Source: CAD feature listing. Evaluate the final solid. Frame: model axes, mm. A direction names the side the tool comes from. Give positions to 0.01 mm unless a question says otherwise; leave off trailing zeros. Write each loop counter-clockwise with the first axis right and the second up, starting at its lowest first coordinate (ties: lowest second). Pieces come first, ordered by that corner, then holes. Notation, with made-up numbers: (9, 66.25) -> (62, 66.25) arc R20 ccw to (62, 98.25) -> close; hole circle Ø9 at (-35.75, 40.25). An arc over 180 degrees is marked (long way). Answer as a JSON object with one key per item and string values. Group by question number.
Item 1: Pull-direction query (X, two-part tool) for faces 4 (the face through (-1.42, -3.92, 0)), 5 (the face through (-0.867, -3.905, 6.902)), 6 (the face through (1, -1, 7)); classes: pulls with the +X half, pulls with the -X half, needs draft (parallel to the pull), parting line crosses it, or undercut.
Item 2: Section query B-B on y = 0. Return the cut outline in (x, z).
Item 3: First-contact query: pin 1 Ø3 at (x, z) = (0, 7.5) entering from -Y; pin 2 Ø6 at (x, z) = (2.5, 7) entering from +Y; pin 3 Ø2 at (x, z) = (-4.5, 11.5) entering from -Y. Flat tips, straight axial feed; report the tip coordinate or a pass-through.
Item 4: Section query A-A on x = 0. Return the cut outline in (y, z).
Item 5: Section query C-C on z = 13.25. Return the cut outline in (x, y).
Item 6: Ray query, probe 1 along Y at (x, z) = (0, 12.5); probe 2 along Y at (x, z) = (-0.5, 10); probe 3 along Z at (x, y) = (3.5, -4). Return the intervals inside material, ascending. Write a range as from..to.
Item 7: Section query D-D on z = 3.5. Return the cut outline in (x, y), plus the area to 3 significant figures.
Item 8: Access query for faces 1 (the face through (4.197, 1.322, 14.394)), 2 (the face through (-0.06, -1.7, 2.94)), 3 (the face through (-0.1, 1.4, -1)). Directions: +Z, -Z, +X, -X, +Y, -Y. A direction counts if a zero-diameter tool reaches every point of the face in a straight line with its end or side. Return the directions, or none.
from build123d import *

# Parameters (mm, degrees)
SKETCH_R             = 4
PAD_DEPTH            = 14
SKETCH001_R          = 4.4
PAD001_DEPTH         = 1.5
CHAMFER_SIZE         = 0.7
SKETCH002_R          = 6
PAD002_DEPTH         = 1
POCKET_DEPTH         = 8
SKETCH004_R          = 1
POCKET001_DEPTH      = 1.001
POCKET001_DEPTH_BACK = -15.501


with BuildPart() as part:
    # Sketch → Pad (new body)
    with BuildSketch(Plane.XY):
        Circle(SKETCH_R)
    extrude(amount=PAD_DEPTH)

    # Sketch001 (on Face3 of Pad) → Pad001 (join)
    with BuildSketch(Plane.XY.offset(14)):
        Circle(SKETCH001_R)
    extrude(amount=PAD001_DEPTH)

    # Chamfer
    chamfer_edges = [part.edges().sort_by_distance(p)[0] for p in [
        (-4.4, 0, 15.5),
    ]]
    chamfer(chamfer_edges, length=CHAMFER_SIZE)

    # Sketch002 → Pad002 (join)
    with BuildSketch(Plane.XY):
        Circle(SKETCH002_R)
    extrude(amount=-PAD002_DEPTH)

    # Sketch003 → Pocket (cut)
    with BuildSketch(Plane.XY.offset(-1)):
        with BuildLine():
            ThreePointArc((-1.204159, 1.2), (0, -1.7), (1.204159, 1.2))
            Line((-1.204159, 1.2), (1.204159, 1.2))
        make_face()
    extrude(amount=POCKET_DEPTH, mode=Mode.SUBTRACT)

    # Sketch004 → Pocket001 (cut, two sides)
    with BuildSketch(Plane.XY) as pocket001_sk:
        Circle(SKETCH004_R)
    extrude(amount=-POCKET001_DEPTH, mode=Mode.SUBTRACT)
    extrude(pocket001_sk.sketch, amount=-POCKET001_DEPTH_BACK, mode=Mode.SUBTRACT)


solid = part.part
Worked answers:
{
 "1": {"face 4": "needs draft", "face 5": "parting line crosses it", "face 6": "undercut"},
 "2": {"outline": "(-6, -1) -> (-1.7, -1) -> (-1.7, 7) -> (-1, 7) -> (-1, 15.5) -> (-3.7, 15.5) -> (-4.4, 14.8) -> (-4.4, 14) -> (-4, 14) -> (-4, 0) -> (-6, 0) -> close; (1, 7) -> (1.7, 7) -> (1.7, -1) -> (6, -1) -> (6, 0) -> (4, 0) -> (4, 14) -> (4.4, 14) -> (4.4, 14.8) -> (3.7, 15.5) -> (1, 15.5) -> close"},
 "3": {"pin 1": "y = -4", "pin 2": "y = 4", "pin 3": "y = -1.94"},
 "4": {"outline": "(-6, -1) -> (-1.7, -1) -> (-1.7, 7) -> (-1, 7) -> (-1, 15.5) -> (-3.7, 15.5) -> (-4.4, 14.8) -> (-4.4, 14) -> (-4, 14) -> (-4, 0) -> (-6, 0) -> close; (1, 7) -> (1.2, 7) -> (1.2, -1) -> (6, -1) -> (6, 0) -> (4, 0) -> (4, 14) -> (4.4, 14) -> (4.4, 14.8) -> (3.7, 15.5) -> (1, 15.5) -> close"},
 "5": {"outline": "circle Ø8 at (0, 0); hole circle Ø2 at (0, 0)"},
 "6": {"probe 1": "-4..-1, 1..4", "probe 2": "-3.97..-0.87, 0.87..3.97", "probe 3": "-1..0"},
 "7": {"outline": "circle Ø8 at (0, 0); hole (-1.2, 1.2) arc R1.7 ccw (long way) to (1.2, 1.2) -> close", "area": "42.0 mm^2"},
 "8": {"face 1": "+Z", "face 2": "-Z", "face 3": "-Z, +X, -X, +Y, -Y"}
}
